```python
from build123d import *

# Parameters (mm, degrees)
ESQUISSE1_W        = 90
ESQUISSE1_H        = 25
ESQUISSE1_R        = 1.75
BOSS_EXTRU_1_DEPTH = 3


with BuildPart() as part:
    # Esquisse1 → Boss.-Extru.1 (new body)
    with BuildSketch(Plane(origin=(0, 0, 0), x_dir=(1, 0, 0), z_dir=(0, 1, 0))):
        Rectangle(ESQUISSE1_W, ESQUISSE1_H)
        with Locations((-41, -1.5)):
            Circle(ESQUISSE1_R, mode=Mode.SUBTRACT)
        with Locations((41, -1.5)):
            Circle(ESQUISSE1_R, mode=Mode.SUBTRACT)
        with Locations((0, -6)):
            Circle(ESQUISSE1_R, mode=Mode.SUBTRACT)
    extrude(amount=BOSS_EXTRU_1_DEPTH)


solid = part.part
```
The model under review builds one solid part; all positions refer to its coordinate system, in mm. Coordinates: 2 decimals unless noted, no trailing zeros. Write each loop counter-clockwise with the first axis right and the second up, starting at its lowest first coordinate (ties: lowest second). Pieces come first, ordered by that corner, then holes. Notation, with made-up numbers: (-28, 11.5) -> (-19, 11.5) arc R22 ccw to (-19, 36.5) -> close; hole circle Ø3 at (-24.75, -19.75). An arc over 180 degrees is marked (long way). One line per item, written item: value. Start each with the question number.
Q1. Add section C-C, the plane z = 6. Give the boundary of the cut face in (x, y), then the cut area to 4 significant figures.
Q2. To check wall thickness, follow probe 1 along X at (y, z) = (1.3, 1.5); probe 2 along X at (y, z) = (1.5, 6); probe 3 along X at (y, z) = (2.1, 0.5). State the ranges of each line that lie inside material, in increasing order.
Q3. The part is to be moulded in two halves that separate along X. For faces 1 (the face through (-0.38, 1.48, 7.71)), 2 (the face through (42.617, 1.479, 2.17)), 3 (the face through (45, 1, 0)), 4 (the face through (-1, 0, 0)), say which applies: +X half, -X half, draft (parallel to the pull), parting line (faces both ways), or undercut.
Q4. Clearance check with a flat-ended pin moving along its axis: P1, Ø3, axis at x = 0, z = 6, coming from the +Y side. State where the tip first meets the part, or that it passes through.
Q5. Add section A-A, the plane x = 0. Give the boundary of the cut face in (y, z), then the cut area to 3 significant figures.
Q6. Add section B-B, the plane z = 1.5. Give the boundary of the cut face in (x, y), then the cut area to 3 significant figures.
Response:
1. outline: (-45, 0) -> (-1.75, 0) -> (-1.75, 3) -> (-45, 3) -> close; (1.75, 0) -> (45, 0) -> (45, 3) -> (1.75, 3) -> close
1. area: 259.5 mm²
2. probe 1: -45 to -42.75, -39.25 to 39.25, 42.75 to 45
2. probe 2: -45 to -1.75, 1.75 to 45
2. probe 3: -45 to -42.44, -39.56 to 39.56, 42.44 to 45
3. face 1: undercut
3. face 2: undercut
3. face 3: +X half
3. face 4: draft
4. P1: through
5. outline: (0, -12.5) -> (3, -12.5) -> (3, 4.25) -> (0, 4.25) -> close; (0, 7.75) -> (3, 7.75) -> (3, 12.5) -> (0, 12.5) -> close
5. area: 64.5 mm²
6. outline: (-45, 0) -> (-42.75, 0) -> (-42.75, 3) -> (-45, 3) -> close; (-39.25, 0) -> (39.25, 0) -> (39.25, 3) -> (-39.25, 3) -> close; (42.75, 0) -> (45, 0) -> (45, 3) -> (42.75, 3) -> close
6. area: 249 mm²
